Here's how the part is built. I have some questions about the finished solid (model axes, mm). A direction names the side the tool comes from. Round coordinates to 2 decimals unless told otherwise and drop trailing zeros. Loops run counter-clockwise (first coordinate to the right, second up) from the corner with the lowest first, then second, coordinate; pieces in that order, holes last. Notation, with made-up numbers: M 3.5,78.25 L 48.5,78.25 A7 cw 48.5,88.25 Z; hole C 19.25,21.5 d1. An arc over 180 degrees is marked long. Answer as CSV lines item,"result".
```python
from build123d import *

# Parameters (mm, degrees)
SKETCH1_W           = 63.5
SKETCH1_H           = 12.7
BOSS_EXTRUDE1_DEPTH = 3.175
SKETCH2_W           = 50.8
SKETCH2_H           = 38.1
BOSS_EXTRUDE2_DEPTH = 3.175
BOSS_EXTRUDE3_DEPTH = 12.7
SKETCH3_R           = 0.79375
CUT_EXTRUDE1_DEPTH  = 6.35
LPATTERN1_COUNT     = 5
LPATTERN1_PITCH     = 3.175
SKETCH5_R           = 0.79375
CUT_EXTRUDE2_DEPTH  = 6.35
LPATTERN2_COUNT     = 5
LPATTERN2_PITCH     = 3.175
SKETCH6_R           = 3.175
CUT_EXTRUDE3_DEPTH  = 54.975


with BuildPart() as part:
    # Sketch1 → Boss-Extrude1 (new body)
    with BuildSketch(Plane.XY):
        Rectangle(SKETCH1_W, SKETCH1_H)
    extrude(amount=BOSS_EXTRUDE1_DEPTH)



with BuildPart() as body_2:
    # Sketch2 → Boss-Extrude2 (new body)
    with BuildSketch(Plane.ZY.offset(31.75)):
        with Locations((-25.4, 0)):
            Rectangle(SKETCH2_W, SKETCH2_H)
    extrude(amount=BOSS_EXTRUDE2_DEPTH)


with BuildPart() as part_1:
    add(part.part)

    add(body_2.part)  # Boss-Extrude3 merges body 2
    # Sketch4 → Boss-Extrude3 (add)
    with BuildSketch(Plane(origin=(0, 6.35, 0), x_dir=(1, 0, 0), z_dir=(0, 1, 0))):
        with BuildLine():
            Line((-34.925, 0), (-31.75, 0))
            Line((-31.75, 0), (-31.75, -3.175))
            ThreePointArc((-31.75, -3.175), (-33.99506403, -2.24506403), (-34.925, 0))
        make_face()
    extrude(amount=-BOSS_EXTRUDE3_DEPTH)

    # Sketch3 → Cut-Extrude1 (cut)
    with BuildSketch(Plane.XY.offset(3.175)):
        with Locations((25.4, 0)):
            Circle(SKETCH3_R)
    cut_extrude1 = extrude(amount=-CUT_EXTRUDE1_DEPTH, mode=Mode.SUBTRACT)

    # LPattern1: Cut-Extrude1 ×5
    with Locations(*[(-i * LPATTERN1_PITCH, 0, 0) for i in range(1, LPATTERN1_COUNT)]):
        add(cut_extrude1, mode=Mode.SUBTRACT)

    # Sketch5 → Cut-Extrude2 (cut)
    with BuildSketch(Plane.XY.offset(3.175)):
        with Locations((-4.7625, 0)):
            Circle(SKETCH5_R)
    cut_extrude2 = extrude(amount=-CUT_EXTRUDE2_DEPTH, mode=Mode.SUBTRACT)

    # LPattern2: Cut-Extrude2 ×5
    with Locations(*[(-i * LPATTERN2_PITCH, 0, 0) for i in range(1, LPATTERN2_COUNT)]):
        add(cut_extrude2, mode=Mode.SUBTRACT)

    # Sketch6 → Cut-Extrude3 (cut, through all)
    with BuildSketch(Plane.XY.offset(3.175)):
        with Locations((3.96875, 0)):
            Circle(SKETCH6_R)
    extrude(amount=-CUT_EXTRUDE3_DEPTH, mode=Mode.SUBTRACT)


solid = part_1.part
```
1. If I drill on line 1 (X direction, y = 14, z = -15.5) (3 decimals); line 2 (Z direction, x = -32, y = -9); line 3 (Z direction, x = -24, y = 1) (3 decimals), over which ranges is the centre line in solid material (lowest first)? Write a range as [from, to].
Evaluation:
line 1,"x = [-34.925, -31.75]"
line 2,"z = [-50.8, 0]"
line 3,"z = [0, 3.175]"
2. I want a section at C-C, the plane z = -13. Please give me the cut outline in (x, y) (3 decimals).
Evaluation:
outline,"M -34.925,-19.05 L -31.75,-19.05 L -31.75,19.05 L -34.925,19.05 Z"
3. I want a section at D-D, the plane y = 8. Please give me the cut outline in (x, z) (3 decimals).
Evaluation:
outline,"M -34.925,-50.8 L -31.75,-50.8 L -31.75,0 L -34.925,0 Z"
4. We'd pull the mould along X, two halves only. Please class faces 4 (the cylindrical face through (-33.97, 0.09, 2.27)), 5 (the flat face through (-31.75, 0, -26)), 6 (the flat face through (-33, -13, 0)), 7 (the cylindrical face through (-10.355, 0.238, 1.61)): pulls with the +X half, pulls with the -X half, needs draft (parallel to the pull), parting line crosses it, or undercut.
Evaluation:
face 4,"pulls with the -X half"
face 5,"pulls with the +X half"
face 6,"needs draft"
face 7,"undercut"
5. For P1, Ø1.6, axis at x = -7.5, z = 1, coming from the +Y side; P2, Ø2.5, axis at x = -32.5, y = 15.5, coming from the +Z side; P3, Ø1.8, axis at x = -11.11, y = 0, coming from the -Z side, each with a flat end and sliding along its axis, tell me the tip position at first contact or that it passes through.
Evaluation:
P1,"stops at y = 6.35"
P2,"stops at z = 0"
P3,"stops at z = 0"
6. I want a section at A-A, the plane x = 12.7. Please give me the cut outline in (y, z) (3 decimals), and give its area (3 significant figures).
Evaluation:
outline,"M -6.35,0 L -0.794,0 L -0.794,3.175 L -6.35,3.175 Z; M 0.794,0 L 6.35,0 L 6.35,3.175 L 0.794,3.175 Z"
area,"35.3 mm²"
7. I want a section at B-B, the plane y = 0. Count the separate pieces of the cut face and the enclosed holes in it, and give its area (3 significant figures).
Evaluation:
separate pieces,"12"
enclosed holes,"0"
area,"300 mm²"
8. Which directions (+Z, -Z, +X, -X, +Y, -Y) give clear straight access to the entire face, cutting with the end or side of a thin tool? Please do faces 1 (the flat face through (0, 0, 0)), 2 (the flat face through (-33, -19.05, -26)), 3 (the flat face through (-33, 13, 0)).
Evaluation:
face 1,"-Z, +X, +Y, -Y"
face 2,"+Z, -Z, +X, -X, -Y"
face 3,"+Z, +X, -X, +Y"
